Source: CAD feature listing. Evaluate the final solid. Frame: model axes, mm. A direction names the side the tool comes from. Round coordinates to 2 decimals unless told otherwise and drop trailing zeros. Write each loop counter-clockwise with the first axis right and the second up, starting at its lowest first coordinate (ties: lowest second). Pieces come first, ordered by that corner, then holes.
from build123d import *

# Parameters (mm, degrees)
SKETCH010_W     = 60
SKETCH010_H     = 5
PAD005_DEPTH    = 22
SKETCH011_W     = 60
SKETCH011_H     = 40
PAD006_DEPTH    = 3
FILLET_R        = 2
FILLET001_R     = 1.4
SKETCH012_R     = 1.4
POCKET005_DEPTH = 15


with BuildPart() as part:
    # Sketch010 → Pad005 (new body)
    with BuildSketch(Plane.XY):
        with Locations((0, 12.5)):
            Rectangle(SKETCH010_W, SKETCH010_H)
    extrude(amount=-PAD005_DEPTH)

    # Sketch011 (on Face6 of Pad005) → Pad006 (join)
    with BuildSketch(Plane(origin=(0, 0, -22), x_dir=(1, 0, 0), z_dir=(0, 0, -1))):
        with Locations((0, 5)):
            Rectangle(SKETCH011_W, SKETCH011_H)
    extrude(amount=PAD006_DEPTH)

    # Fillet
    fillet_edges = [part.edges().sort_by_distance(p)[0] for p in [
        (0, 15, -25),
    ]]
    fillet(fillet_edges, radius=FILLET_R)

    # Fillet001
    fillet001_edges = [part.edges().sort_by_distance(p)[0] for p in [
        (30, -25, -23.5),
        (-30, -25, -23.5),
        (0, -25, -22),
        (0, -25, -25),
    ]]
    fillet(fillet001_edges, radius=FILLET001_R)

    # Sketch012 (on Face14 of Fillet001) → Pocket005 (cut)
    with BuildSketch(Plane.XY):
        with Locations((-20, 12.5)):
            Circle(SKETCH012_R)
        with Locations((0, 12.5)):
            Circle(SKETCH012_R)
        with Locations((20, 12.5)):
            Circle(SKETCH012_R)
    extrude(amount=-POCKET005_DEPTH, mode=Mode.SUBTRACT)


solid = part.part
1) Section query D-D on x = -12.5. Return the cut outline in (y, z).
Taken from the geometry:
outline: (-25, -23.6) arc R1.4 ccw to (-23.6, -25) - (13, -25) arc R2 ccw to (15, -23) - (15, 0) - (10, 0) - (10, -22) - (-23.6, -22) arc R1.4 ccw to (-25, -23.4) - close
2) Section query B-B on z = -6.75. Return the cut outline in (x, y), then the cut area to 3 significant figures.
Taken from the geometry:
outline: (-30, 10) - (30, 10) - (30, 15) - (-30, 15) - close; hole circle Ø2.8 at (-20, 12.5); hole circle Ø2.8 at (0, 12.5); hole circle Ø2.8 at (20, 12.5)
area: 282 mm2
3) Contact query for flat-ended pins moving along their axis: P1, Ø2, axis at x = 20, y = 12.5, coming from the +Z side; P2, Ø2, axis at y = 8, z = -6, coming from the +X side. Output: stop coordinate, or through.
Taken from the geometry:
P1: stops at z = -15
P2: passes through
4) Section query C-C on y = -17.5. Return the cut outline in (x, z).
Taken from the geometry:
outline: (-30, -25) - (30, -25) - (30, -22) - (-30, -22) - close
5) Reachability of faces 1 (the face through (0, -7, -22)), 2 (the face through (0.75, 13.68, -7.4)), 3 (the face through (29.738, -24.416, -23.521)) from +Z, -Z, +X, -X, +Y, -Y: full face, straight path, thin tool, end or side. Return the list, or none.
Taken from the geometry:
face 1: +Z, +X, -X, -Y
face 2: +Z
face 3: +Z, -Z, +X, -Y
6) Pull-direction query (X, two-part tool) for faces 4 (the face through (0.42, 14.43, -24.4)), 5 (the face through (-20, 13, -15)), 6 (the face through (30, 3, -23)); classes: released by +X, released by -X, zero draft, split by the parting line, or undercut.
Taken from the geometry:
face 4: zero draft
face 5: undercut
face 6: released by +X
7) Section query A-A on x = -20. Return the cut outline in (y, z), then the cut area to 3 significant figures.
Taken from the geometry:
outline: (-25, -23.6) arc R1.4 ccw to (-23.6, -25) - (13, -25) arc R2 ccw to (15, -23) - (15, 0) - (13.9, 0) - (13.9, -15) - (11.1, -15) - (11.1, 0) - (10, 0) - (10, -22) - (-23.6, -22) arc R1.4 ccw to (-25, -23.4) - close
area: 186 mm2
8) Material intervals for line 1 (Y direction, x = -20, z = -3.75); line 2 (Z direction, x = 13, y = -9); line 3 (Y direction, x = -23, z = -19.5), sorted ascending.
Taken from the geometry:
line 1: y = 10 to 11.1, 13.9 to 15
line 2: z = -25 to -22
line 3: y = 10 to 15
